Geometry: final body of the model. Coordinates: model frame, mm. Coordinates: 2 decimals unless noted, no trailing zeros. Loops run counter-clockwise (first coordinate to the right, second up) from the corner with the lowest first, then second, coordinate; pieces in that order, holes last. Notation, with made-up numbers: (27.25, 71) - (42.25, 71) arc R26 ccw to (42.25, 93) - close; hole circle Ø10 at (-13, 41.25). An arc over 180 degrees is marked (long way). Return JSON: item names as keys, results as strings.
from build123d import *

# Parameters (mm, degrees)
SKETCH1_R                                 = 3
BOSS_EXTRUDE1_DEPTH                       = 275
SKETCH3_W                                 = 0.8
SKETCH3_H                                 = 0.5
CUT_EXTRUDE2_DEPTH                        = 276.032725326
CUT_EXTRUDE2_DEPTH_BACK                   = 276.032725326
SKETCH4_W                                 = 3.470061058
SKETCH4_H                                 = 7
SKETCH4_W_2                               = 2.92528695
CHAMFER1_SIZE                             = 0.3
RETAINING_GROOVES_D5P7_1_START            = 7.05
SKETCH5_R                                 = 2.85
SKETCH5_R_2                               = 2.49
RETAINING_GROOVES_D5P7_1_DEPTH            = 0.8
RETAINING_GROOVES_D5P7_2_START            = 13
SKETCH6_R                                 = 2.85
SKETCH6_R_2                               = 2.49
RETAINING_GROOVES_D5P7_2_DEPTH            = 0.8
RETAINING_GROOVES_D5P7_3_START            = 260.25
SKETCH7_R                                 = 2.85
SKETCH7_R_2                               = 2.49
RETAINING_GROOVES_D5P7_3_DEPTH            = 0.8
RETAINING_GROOVES_D5P7_4_START            = 266.2
SKETCH8_R                                 = 2.85
SKETCH8_R_2                               = 2.49
RETAINING_GROOVES_D5P7_4_DEPTH            = 0.8
TWO_HUB_CROSS_PIN_D2_DEPTH                = 276.032725326
TWO_HUB_CROSS_PIN_D2_DEPTH_BACK           = 276.032725326
SKETCH9_R                                 = 1
SKETCH10_R                                = 3.1
REVB_LOWER_SHAFT_NOSE_CLEARANCE_2MM_DEPTH = 2


with BuildPart() as part:
    # Sketch1 → Boss-Extrude1 (new body)
    with BuildSketch(Plane.XY):
        Circle(SKETCH1_R)
    extrude(amount=BOSS_EXTRUDE1_DEPTH)

    # Sketch3 → Cut-Revolve1 (revolve, cut)
    with BuildSketch(Plane(origin=(0, 0, 0), x_dir=(0, 0, -1), z_dir=(1, 0, 0)), mode=Mode.PRIVATE) as cut_revolve1_sk:
        with Locations((-266.6, 2.75)):
            Rectangle(SKETCH3_W, SKETCH3_H)
        with Locations((-260.65, 2.75)):
            Rectangle(SKETCH3_W, SKETCH3_H)
        with Locations((-13.4, 2.75)):
            Rectangle(SKETCH3_W, SKETCH3_H)
        with Locations((-7.45, 2.75)):
            Rectangle(SKETCH3_W, SKETCH3_H)
    revolve(cut_revolve1_sk.sketch.rotate(Axis((0, 0, 263.365004794), (0, 0, -1)), 90), axis=Axis((0, 0, 263.365004794), (0, 0, -1)), mode=Mode.SUBTRACT)

    # Sketch4 → Cut-Extrude2 (cut, two sides: drawn at the far end of the back side and taken through both)
    with BuildSketch(Plane(origin=(0, 0, 0), x_dir=(1, 0, 0), z_dir=(0, 1, 0)).offset(-CUT_EXTRUDE2_DEPTH_BACK)):
        with Locations((4.235030529, -3.5)):
            Rectangle(SKETCH4_W, SKETCH4_H)
        with Locations((-3.962643475, -3.5)):
            Rectangle(SKETCH4_W_2, SKETCH4_H)
    extrude(amount=CUT_EXTRUDE2_DEPTH + CUT_EXTRUDE2_DEPTH_BACK, mode=Mode.SUBTRACT)

    # Chamfer1
    chamfer1_edges = [part.edges().sort_by_distance(p)[0] for p in [
        (0, 3, 0),
        (0, -3, 0),
    ]]
    chamfer(chamfer1_edges, length=CHAMFER1_SIZE)

    # Sketch5 → Retaining_Grooves_D5p7_1 (add)
    with BuildSketch(Plane.XY.offset(RETAINING_GROOVES_D5P7_1_START)):
        Circle(SKETCH5_R)
        Circle(SKETCH5_R_2, mode=Mode.SUBTRACT)
    extrude(amount=RETAINING_GROOVES_D5P7_1_DEPTH)

    # Sketch6 → Retaining_Grooves_D5p7_2 (add)
    with BuildSketch(Plane.XY.offset(RETAINING_GROOVES_D5P7_2_START)):
        Circle(SKETCH6_R)
        Circle(SKETCH6_R_2, mode=Mode.SUBTRACT)
    extrude(amount=RETAINING_GROOVES_D5P7_2_DEPTH)

    # Sketch7 → Retaining_Grooves_D5p7_3 (add)
    with BuildSketch(Plane.XY.offset(RETAINING_GROOVES_D5P7_3_START)):
        Circle(SKETCH7_R)
        Circle(SKETCH7_R_2, mode=Mode.SUBTRACT)
    extrude(amount=RETAINING_GROOVES_D5P7_3_DEPTH)

    # Sketch8 → Retaining_Grooves_D5p7_4 (add)
    with BuildSketch(Plane.XY.offset(RETAINING_GROOVES_D5P7_4_START)):
        Circle(SKETCH8_R)
        Circle(SKETCH8_R_2, mode=Mode.SUBTRACT)
    extrude(amount=RETAINING_GROOVES_D5P7_4_DEPTH)

    # Sketch9 → Two_Hub_Cross_Pin_D2 (cut, two sides: drawn at the far end of the back side and taken through both)
    with BuildSketch(Plane(origin=(0, 0, 0), x_dir=(0, 0, -1), z_dir=(1, 0, 0)).offset(-TWO_HUB_CROSS_PIN_D2_DEPTH_BACK)):
        with Locations((-41.5, 0)):
            Circle(SKETCH9_R)
        with Locations((-243.5, 0)):
            Circle(SKETCH9_R)
    extrude(amount=TWO_HUB_CROSS_PIN_D2_DEPTH + TWO_HUB_CROSS_PIN_D2_DEPTH_BACK, mode=Mode.SUBTRACT)

    # Sketch10 → RevB_Lower_Shaft_Nose_Clearance_2mm (cut)
    with BuildSketch(Plane(origin=(0, 0, 0), x_dir=(-1, 0, 0), z_dir=(0, 0, -1))):
        Circle(SKETCH10_R)
    extrude(amount=-REVB_LOWER_SHAFT_NOSE_CLEARANCE_2MM_DEPTH, mode=Mode.SUBTRACT)


solid = part.part
Item 1: Section query A-A, the plane y = 0. Count the separate pieces of the cut face and the enclosed holes in it, and give its area (3 significant figures).
Worked out:
{"separate pieces": "3", "enclosed holes": "0", "area": "1,610 mm^2"}
Item 2: Ray query, probe 1 along Z at (x, y) = (1.5, 0); probe 2 along Y at (x, z) = (1, 41.5); probe 3 along Z at (x, y) = (-1.75, -0.5). Return the intervals inside material, ascending. Write a range as from..to.
Worked out:
{"probe 1": "2..40.5, 42.5..242.5, 244.5..275", "probe 2": "-2.83..-1, 1..2.83", "probe 3": "2..40.63, 42.37..242.63, 244.37..275"}
Item 3: Section query B-B, the plane z = 158. Return loops of the section in (x, y), and give its area (3 significant figures).
Worked out:
{"outline": "circle Ø6 at (0, 0)", "area": "28.3 mm^2"}
Item 4: First-contact query: pin 1 Ø1.7 at (y, z) = (0, 3.5) entering from -X; pin 2 Ø0.6 at (x, y) = (3, 0.5) entering from -Z; pin 3 Ø1 at (y, z) = (0.5, 5) entering from +X. Flat tips, straight axial feed; report the tip coordinate or a pass-through.
Worked out:
{"pin 1": "x = -2.5", "pin 2": "z = 7", "pin 3": "x = 2.5"}
